```python
from build123d import *

# Parameters (mm, degrees)
SKETCH3_W              = 38.2050925
SKETCH3_H              = 0.551638054
BOSS_EXTRUDE1_DEPTH    = 46.736
CUT_EXTRUDE1_START     = -17.483231481
CUT_EXTRUDE1_OUTLINE_R = 2.200841193
CUT_EXTRUDE1_DEPTH     = 34.966462962
SCALE1_SCALE           = 2.1025641


# Read off the part's stored shape, not the designer's step: Cut-Extrude1
with BuildPart() as part:
    # Sketch3 → Revolve1 (revolve)
    with BuildSketch(Plane.XY, mode=Mode.PRIVATE) as revolve1_sk:
        with Locations((-176.077749649, -229.697714421)):
            Rectangle(SKETCH3_W, SKETCH3_H)
    revolve(revolve1_sk.sketch.rotate(Axis((-195.180295899, -229.973533448, 0), (0, 1, 0)), 90), axis=Axis((-195.180295899, -229.973533448, 0), (0, 1, 0)))

    # Sketch4 → Boss-Extrude1 (add)
    with BuildSketch(Plane.XZ.offset(229.973533448)):
        with BuildLine():
            Line((-209.32977738, -17.483231481), (-181.030814417, -17.483231481))
            ThreePointArc((-181.030814417, -17.483231481), (-178.673497186, -16.506798713), (-177.697064417, -14.149481481))
            Line((-177.697064417, -14.149481481), (-177.697064417, 14.149481481))
            ThreePointArc((-177.697064417, 14.149481481), (-178.673497186, 16.506798713), (-181.030814417, 17.483231481))
            Line((-181.030814417, 17.483231481), (-209.32977738, 17.483231481))
            ThreePointArc((-209.32977738, 17.483231481), (-211.687094612, 16.506798713), (-212.66352738, 14.149481481))
            Line((-212.66352738, 14.149481481), (-212.66352738, -14.149481481))
            ThreePointArc((-212.66352738, -14.149481481), (-211.687094612, -16.506798713), (-209.32977738, -17.483231481))
        make_face()
        with BuildLine():
            Line((-211.07602738, -13.355731481), (-211.07602738, 13.355731481))
            ThreePointArc((-211.07602738, 13.355731481), (-210.332078604, 15.151782705), (-208.53602738, 15.895731481))
            Line((-208.53602738, 15.895731481), (-181.824564417, 15.895731481))
            ThreePointArc((-181.824564417, 15.895731481), (-180.028513193, 15.151782705), (-179.284564417, 13.355731481))
            Line((-179.284564417, 13.355731481), (-179.284564417, -13.355731481))
            ThreePointArc((-179.284564417, -13.355731481), (-180.028513193, -15.151782705), (-181.824564417, -15.895731481))
            Line((-181.824564417, -15.895731481), (-208.53602738, -15.895731481))
            ThreePointArc((-208.53602738, -15.895731481), (-210.332078604, -15.151782705), (-211.07602738, -13.355731481))
        make_face(mode=Mode.SUBTRACT)
    extrude(amount=BOSS_EXTRUDE1_DEPTH)

    # Cut-Extrude1 outline → Cut-Extrude1 (cut)
    with BuildSketch(Plane.XY.offset(CUT_EXTRUDE1_START)):
        with Locations((-205.51977738, -239.498533448)):
            Circle(CUT_EXTRUDE1_OUTLINE_R)
        with BuildLine():
            ThreePointArc((-196.813996528, -239.864188004), (-195.14024192, -246.930599786), (-193.618948859, -239.82980424))
            Line((-193.618948859, -239.82980424), (-193.618948859, -235.096274088))
            Line((-193.618948859, -235.096274088), (-196.813996528, -235.096274088))
            Line((-196.813996528, -235.096274088), (-196.813996528, -239.864188004))
        make_face()
        with BuildLine():
            ThreePointArc((-196.813996528, -267.015063616), (-195.14024192, -274.081475398), (-193.618948859, -266.980679852))
            Line((-193.618948859, -266.980679852), (-193.618948859, -262.2471497))
            Line((-193.618948859, -262.2471497), (-196.813996528, -262.2471497))
            Line((-196.813996528, -262.2471497), (-196.813996528, -267.015063616))
        make_face()
        with Locations((-184.840814417, -239.498533448)):
            Circle(CUT_EXTRUDE1_OUTLINE_R)
        with Locations((-205.51977738, -270.359533448)):
            Circle(CUT_EXTRUDE1_OUTLINE_R)
        with Locations((-184.840814417, -270.359533448)):
            Circle(CUT_EXTRUDE1_OUTLINE_R)
    extrude(amount=CUT_EXTRUDE1_DEPTH, mode=Mode.SUBTRACT)


with BuildPart() as part_1:
    # Scale1: scaled about (0, 0, 0)
    add(part.part.scale(SCALE1_SCALE))


solid = part_1.part
```
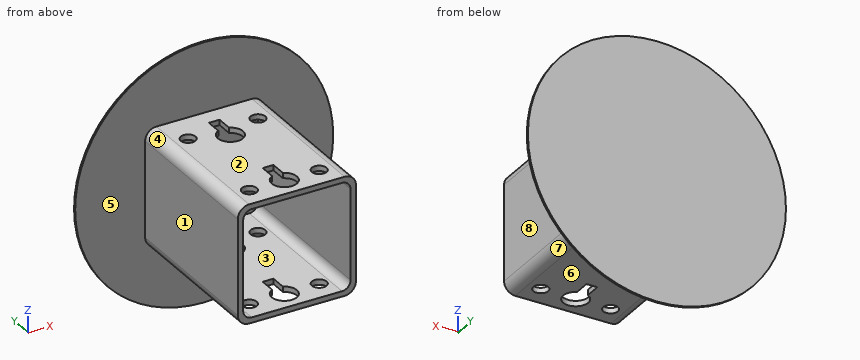
CAD build for the part. Positions are in the model's coordinates, mm. Face numbers are marked on the shaded views. A direction names the side the tool comes from. Coordinates: 2 decimals unless noted, no trailing zeros. Order: outer loops, then holes, each group sorted by start corner. A loop starts at its lowest first (then second) coordinate and runs counter-clockwise, first axis right, second up. Notation, with made-up numbers: (1.25, 54) - (7.25, 54) arc R25 cw to (7.25, 85) - close; hole circle Ø1 at (0, 76.25). An arc over 180 degrees is marked (long way). Use a Markdown table: item, result. Add a question column.
(1) Saw through at A-A (y = -522). Give the cut face in (x, z).
(2) Saw through at B-B (z = 0). Give the cut face in (x, y), then the cut area to 3 significant figures.
(3) Saw through at C-C (x = -395.5). Give the cut face in (y, z), then the cut area to 3 significant figures.
(4) Drill centre lines: line 1 along Z through (x, y) = (-415, -532.5); line 2 along X through (y, z) = (-510.5, -18); line 3 along Y through (x, z) = (-384, 27). Where is each one in solid material? Low to high. Write a range as [from, to].
(5) Saw through at D-D (x = -466.5). Give the cut face in (y, z).
(6) Pull direction X, two halves, no side cores. Call the marked faces 1, 2 and 3: +X half, -X half, draft (parallel to the pull), parting line (faces both ways), or undercut.
(7) Flat gauge pins, fed straight in: pin 1 (8 mm diameter, centred on x = -445, y = -540.5, fed in from -Z); pin 2 (1.7 mm diameter, centred on y = -555.5, z = -34.5, fed in from -X); pin 3 (2.5 mm diameter, centred on y = -498.5, z = 35.5, fed in from +X). Where does each tip first touch, or does it go through?
(8) Which spindle directions (+Z, -Z, +X, -X, +Y, -Y) get a long thin tool onto all of the face, cutting with end or side? Do the marked faces 4, 5, 6, 7 and 8. Say none if no direction does.
Solved:
| question | item | result |
|---|---|---|
| 1 | outline | (-447.14, -29.75) arc R7.01 ccw to (-440.13, -36.76) - (-380.63, -36.76) arc R7.01 ccw to (-373.62, -29.75) - (-373.62, 29.75) arc R7.01 ccw to (-380.63, 36.76) - (-440.13, 36.76) arc R7.01 ccw to (-447.14, 29.75) - close; hole (-443.8, -28.08) arc R5.34 ccw to (-438.46, -33.42) - (-382.3, -33.42) arc R5.34 ccw to (-376.96, -28.08) - (-376.96, 28.08) arc R5.34 ccw to (-382.3, 33.42) - (-438.46, 33.42) arc R5.34 ccw to (-443.8, 28.08) - close |
| 2 | outline | (-490.71, -483.53) - (-447.14, -483.53) - (-447.14, -581.8) - (-443.8, -581.8) - (-443.8, -483.53) - (-376.96, -483.53) - (-376.96, -581.8) - (-373.62, -581.8) - (-373.62, -483.53) - (-330.05, -483.53) - (-330.05, -482.37) - (-490.71, -482.37) - close |
| 2 | area | 842 mm² |
| 3 | outline | (-581.8, -36.76) - (-483.53, -36.76) - (-483.53, -78.94) - (-482.37, -78.94) - (-482.37, 78.94) - (-483.53, 78.94) - (-483.53, 36.76) - (-581.8, 36.76) - (-581.8, 33.42) - (-483.53, 33.42) - (-483.53, -33.42) - (-581.8, -33.42) - close |
| 3 | area | 839 mm² |
| 4 | line 1 | z = [-36.76, -33.42], [33.42, 36.76] |
| 4 | line 2 | x = [-447.14, -443.8], [-376.96, -373.62] |
| 4 | line 3 | y = [-483.53, -482.37] |
| 5 | outline | (-483.53, -57.47) - (-482.37, -57.47) - (-482.37, 57.47) - (-483.53, 57.47) - close |
| 6 | face 1 | -X half |
| 6 | face 2 | draft |
| 6 | face 3 | undercut |
| 7 | pin 1 | stops at z = -36.71 |
| 7 | pin 2 | stops at x = -445.95 |
| 7 | pin 3 | stops at x = -375.25 |
| 8 | face 4 | +Z, -X, -Y |
| 8 | face 5 | -Y |
| 8 | face 6 | -Z, +X, -X, -Y |
| 8 | face 7 | -Z, +X, -Y |
| 8 | face 8 | +Z, -Z, +X, -Y |
